For this review, take the finished solid that the model builds, in its own axes (mm). A direction names the side the tool comes from. Give positions to 0.01 mm unless a question says otherwise; leave off trailing zeros. Order: outer loops, then holes, each group sorted by start corner. A loop starts at its lowest first (then second) coordinate and runs counter-clockwise, first axis right, second up.
Item 1: For probe 1 along X at (y, z) = (5, 19.5); probe 2 along X at (y, z) = (31, 20.25); probe 3 along Z at (x, y) = (12, 40.5), list the stretches that pass through material, from the lowest coordinate up.
Item 2: Machinability: for faces 1 (the flat face through (-12, 4, 10.16)), 2 (the cylindrical face through (12.177, 26.928, 17.673)), 3 (the flat face through (-42.611, 13, 18)), 4 (the cylindrical face through (-11.925, 32.254, 12.878)), 5 (the flat face through (-41, 25.4, 18)), which of the approach directions +Z, -Z, +X, -X, +Y, -Y give a long, thin tool a straight path to every point of the face, cutting with its end or side? Answer none if there is none.
Item 3: Consider section B-B (z = 19.5). Give the boundary of the cut face in (x, y), plus the area to 3 significant figures.
Item 4: For P1, Ø4.5, axis at y = 13, z = 16, coming from the -X side; P2, Ø13, axis at x = -44, y = 32.5, coming from the +Z side; P3, Ø3, axis at x = -40.5, z = 20.5, coming from the +Y side; P4, Ø1.5, axis at y = 38, z = 10.5, coming from the -X side, all flat-tipped, find the tip position at first contact; note any pin that passes through.
Item 5: Consider section D-D (x = -11.5). Give the boundary of the cut face in (y, z), plus the area to 3 significant figures.
Item 6: Consider section A-A (y = 42.5). Give the boundary of the cut face in (x, z).
Item 7: Consider section C-C (y = 14). Give the boundary of the cut face in (x, z), plus the area to 3 significant figures.
Item 8: The part is to be moulded in two halves that separate along X. For faces 6 (the flat face through (-13, 20, 0)), 7 (the flat face through (18.349, 13, 18)), 8 (the flat face through (-50.231, 23, 5)), 9 (the flat face through (-12, 7.62, 18)), say which applies: released by +X, released by -X, zero draft, split by the parting line, or undercut.
```python
from build123d import *

# Parameters (mm, degrees)
F0_W     = 76.2
F0_H     = 50.8
F1_DEPTH = 10.16
F2_W     = 60.96
F2_H     = 50.8
F3_DEPTH = 25.4
F5_DEPTH = 25.401
F4_W     = 8.5195787251
F4_H     = 25.4
F4_W_2   = 7.62
F4_W_3   = 45.72
F4_H_2   = 7.62
F6_DEPTH = 15.24
F7_R     = 5.08
F8_R     = 5.08
F9_R     = 5.08


with BuildPart() as f1:
    # F0 (on Top) → F1 (new body)
    with BuildSketch(Plane.XY):
        with Locations((-12.131340879, 25.4)):
            Rectangle(F0_W, F0_H)
    extrude(amount=F1_DEPTH)

    # F2 (on Top) → F3 (join)
    with BuildSketch(Plane.XY):
        with Locations((-12.131340879, 25.4)):
            Rectangle(F2_W, F2_H)
    extrude(amount=F3_DEPTH)

    # F4 (on face) → F5 (cut, through all)
    with BuildSketch(Plane.XY.offset(25.4)):
        with BuildLine():
            Line((7.5301669641, 50.8), (-30.5567246034, 50.8))
            ThreePointArc((-30.5567246034, 50.8), (-11.5132788196, 32.2496725738), (7.5301669641, 50.8))
        make_face()
        with BuildLine():
            ThreePointArc((7.5367211804, 51.2996725738), (-11.7631365985, 70.3480339493), (-30.5567246034, 50.8))
            Line((-30.5567246034, 50.8), (7.5301669641, 50.8))
            ThreePointArc((7.5301669641, 50.8), (7.5350825558, 51.0498147949), (7.5367211804, 51.2996725738))
        make_face()
    extrude(amount=-F5_DEPTH, mode=Mode.SUBTRACT)

    # F4 (on face) → F6 (cut, through all)
    with BuildSketch(Plane.XY.offset(25.4)):
        with Locations((-38.3515515165, 38.1)):
            Rectangle(F4_W, F4_H)
        with Locations((14.538659121, 38.1)):
            Rectangle(F4_W_2, F4_H)
        with Locations((-12.131340879, 3.81)):
            Rectangle(F4_W_3, F4_H_2)
    extrude(amount=-F6_DEPTH, mode=Mode.SUBTRACT)

    # F7
    f7_edges = [f1.edges().sort_by_distance(p)[0] for p in [
        (-50.231341, 50.8, 5.08),
    ]]
    fillet(f7_edges, radius=F7_R)

    # F8
    f8_edges = [f1.edges().sort_by_distance(p)[0] for p in [
        (25.968659, 50.8, 5.08),
    ]]
    fillet(f8_edges, radius=F8_R)

    # F9
    f9_edges = [f1.edges().sort_by_distance(p)[0] for p in [
        (-34.091762, 25.4, 17.78),
        (10.728659, 25.4, 17.78),
    ]]
    fillet(f9_edges, radius=F9_R)


solid = f1.part
```
Resolved:
1. probe 1: x = -42.61 to -34.99, 10.73 to 18.35
1. probe 2: x = -34.09 to 10.73
1. probe 3: z = 0 to 10.16
2. face 1: +Z, -Y
2. face 2: +Z, +X, +Y
2. face 3: +Z, -X, +Y, -Y
2. face 4: +Z, -Z, +Y
2. face 5: +Z, -X, +Y
3. outline: (-42.61, 0) - (-34.99, 0) - (-34.99, 7.62) - (10.73, 7.62) - (10.73, 0) - (18.35, 0) - (18.35, 25.4) - (15.81, 25.4) arc R5.08 cw to (10.73, 30.48) - (10.73, 50.8) - (7.53, 50.8) arc R19.05 cw to (-30.56, 50.8) - (-34.09, 50.8) - (-34.09, 30.48) arc R5.08 cw to (-39.17, 25.4) - (-42.61, 25.4) - close
3. area: 1,800 mm2
4. P1: stops at x = -42.61
4. P2: stops at z = 10.16
4. P3: stops at y = 25.4
4. P4: stops at x = -50.23
5. outline: (0, 0) - (32.25, 0) - (32.25, 25.4) - (7.62, 25.4) - (7.62, 10.16) - (0, 10.16) - close
5. area: 703 mm2
6. outline: (-50.23, 0) - (-28.41, 0) - (-28.41, 25.4) - (-34.09, 25.4) - (-34.09, 10.16) - (-50.23, 10.16) - close; (5.38, 0) - (25.97, 0) - (25.97, 10.16) - (10.73, 10.16) - (10.73, 25.4) - (5.38, 25.4) - close
7. outline: (-50.23, 0) - (25.97, 0) - (25.97, 10.16) - (18.35, 10.16) - (18.35, 25.4) - (-42.61, 25.4) - (-42.61, 10.16) - (-50.23, 10.16) - close
7. area: 1,700 mm2
8. face 6: zero draft
8. face 7: released by +X
8. face 8: released by -X
8. face 9: undercut
